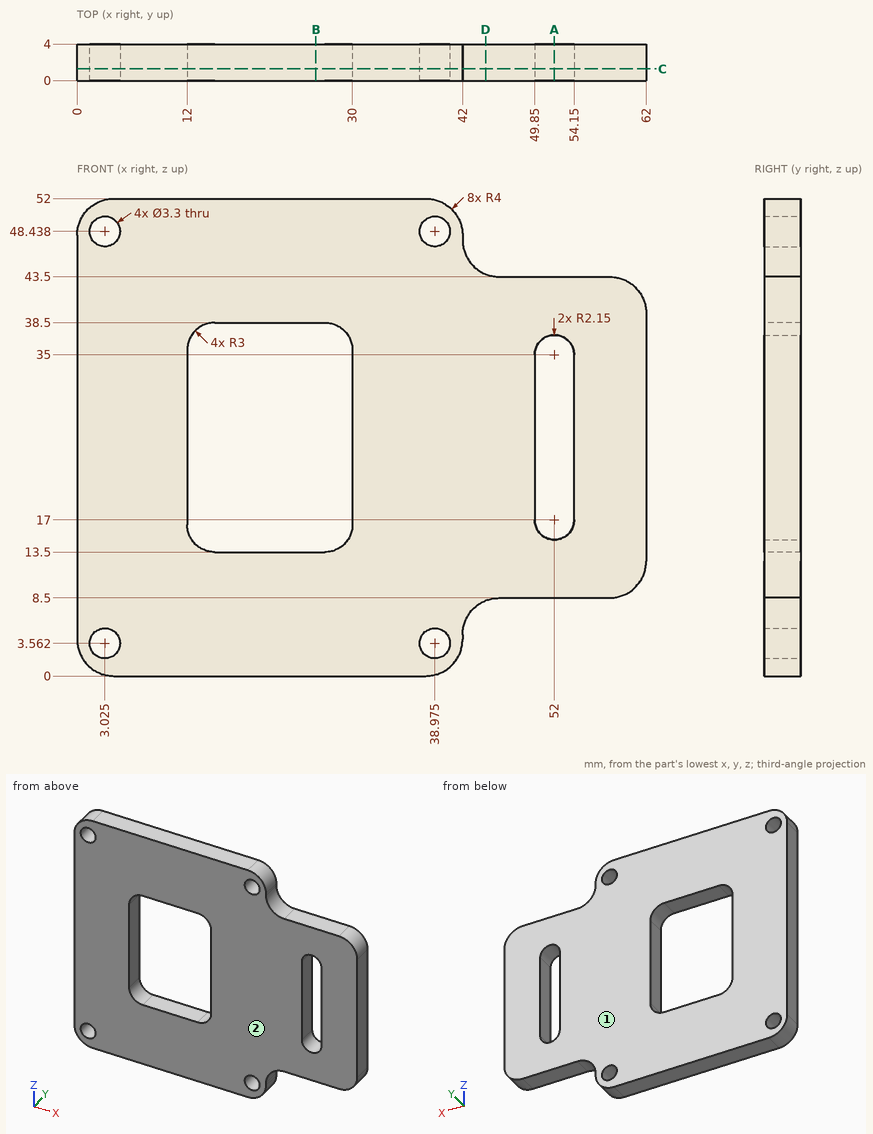
Here's the drawing with two shaded views (mm, measured from the low corner). I have some questions. Coordinates: 2 decimals unless noted, no trailing zeros. Loops run counter-clockwise (first coordinate to the right, second up) from the corner with the lowest first, then second, coordinate; pieces in that order, holes last. Notation, with made-up numbers: (-36.75, 57) -> (-7.75, 57) arc R30 ccw to (-7.75, 81) -> close; hole circle Ø3 at (66.25, -11.75). An arc over 180 degrees is marked (long way). Use one line per item in the form item = value. Start each with the question number.
(1) If we section it at C-C (y = 1.3): Give the number of separate pieces and of enclosed holes in the cut face, then the cut area to 3 significant figures.
(2) Please list where these lines run through material, in increasing order: line 1 along X through (y, z) = (0.6, 29); line 2 along Z through (x, y) = (25.5, 0.9); line 3 along Z through (x, y) = (52, 1.6).
(3) If we section it at A-A (x = 52): Please give me the cut outline in (y, z).
(4) If we section it at D-D (x = 44.5): Please give me the cut outline in (y, z).
(5) If we section it at B-B (x = 26): Please give me the cut outline in (y, z).
(6) We'd pull the mould along Y, two halves only. Please class the marked faces 1 and 2: pulls with the +Y half, pulls with the -Y half, needs draft (parallel to the pull), parting line crosses it, or undercut.
(7) Will these pins go through, and if not, where does the flat tip stop? pin 1 (1.2 mm diameter, centred on x = 52.5, y = 2.5, fed in from +Z); pin 2 (2 mm diameter, centred on x = 50, y = 2.5, fed in from -Z); pin 3 (1.5 mm diameter, centred on y = 2.5, z = 9.5, fed in from +X).
Verdict:
q1.separate_pieces = 1
q1.enclosed_holes = 6
q1.area = 2,300 mm²
q2.line_1 = 0 to 12, 30 to 49.85, 54.15 to 62
q2.line_2 = 0 to 13.5, 38.5 to 52
q2.line_3 = 8.5 to 14.85, 37.15 to 43.5
q3.outline = (0, 8.5) -> (4, 8.5) -> (4, 14.85) -> (0, 14.85) -> close; (0, 37.15) -> (4, 37.15) -> (4, 43.5) -> (0, 43.5) -> close
q4.outline = (0, 8.21) -> (4, 8.21) -> (4, 43.79) -> (0, 43.79) -> close
q5.outline = (0, 0) -> (4, 0) -> (4, 13.5) -> (0, 13.5) -> close; (0, 38.5) -> (4, 38.5) -> (4, 52) -> (0, 52) -> close
q6.face_1 = pulls with the +Y half
q6.face_2 = pulls with the -Y half
q7.pin_1 = 43.5
q7.pin_2 = 8.5
q7.pin_3 = 61.31
